```python
from build123d import *

# Parameters (mm, degrees)
F0_W     = 812.8
F0_H     = 2463.8
F1_DEPTH = 44.45
F3_D     = 228.6
F4_W     = 812.8
F4_H     = 50.8
F5_DEPTH = 3.429


# Not quite as in the source:
# - a feature names something its author has since deleted; it is built from what else it names


with BuildPart() as f1:
    # F0 (on Top) → F1 (new body)
    with BuildSketch(Plane.XY):
        with Locations((406.4, 1231.9)):
            Rectangle(F0_W, F0_H)
    extrude(amount=F1_DEPTH)

    # F3 (through all)
    with Locations(Plane.XY.offset(44.45)):
        with Locations((406.4, 1524)):
            Hole(F3_D / 2)

    # F4 (on face) → F5 (join)
    with BuildSketch(Plane.XY.offset(44.45)):
        with Locations((406.4, 2133.6)):
            Rectangle(F4_W, F4_H)
        with Locations((406.4, 2032)):
            Rectangle(F4_W, F4_H)
        with Locations((406.4, 1930.4)):
            Rectangle(F4_W, F4_H)
        with Locations((406.4, 1828.8)):
            Rectangle(F4_W, F4_H)
        with Locations((406.4, 1727.2)):
            Rectangle(F4_W, F4_H)
        with BuildLine():
            Line((0, 1549.4), (0, 1498.6))
            Line((0, 1498.6), (256.1315735093, 1498.6))
            ThreePointArc((256.1315735093, 1498.6), (254, 1524), (256.1315735093, 1549.4))
            Line((256.1315735093, 1549.4), (0, 1549.4))
        make_face()
        with BuildLine():
            Line((556.6684264907, 1498.6), (812.8, 1498.6))
            Line((812.8, 1498.6), (812.8, 1549.4))
            Line((812.8, 1549.4), (556.6684264907, 1549.4))
            ThreePointArc((556.6684264907, 1549.4), (558.2661716729, 1536.7446420666), (558.8, 1524))
            ThreePointArc((558.8, 1524), (558.2661716729, 1511.2553579334), (556.6684264907, 1498.6))
        make_face()
        with BuildLine():
            Line((490.642269675, 1397), (812.8, 1397))
            Line((812.8, 1397), (812.8, 1447.8))
            Line((812.8, 1447.8), (538.3822715367, 1447.8))
            ThreePointArc((538.3822715367, 1447.8), (517.455945611, 1419.6336407436), (490.642269675, 1397))
        make_face()
        with Locations((406.4, 1320.8)):
            Rectangle(F4_W, F4_H)
        Polygon((0, 1231.9), (0, 1193.8), (812.8, 1193.8), (812.8, 1231.9), (812.8, 1244.6), (0, 1244.6), align=None)
        with Locations((406.4, 1117.6)):
            Rectangle(F4_W, F4_H)
        with Locations((406.4, 1016)):
            Rectangle(F4_W, F4_H)
        with Locations((406.4, 914.4)):
            Rectangle(F4_W, F4_H)
        with Locations((406.4, 812.8)):
            Rectangle(F4_W, F4_H)
        with Locations((406.4, 711.2)):
            Rectangle(F4_W, F4_H)
        with Locations((406.4, 609.6)):
            Rectangle(F4_W, F4_H)
        with Locations((406.4, 508)):
            Rectangle(F4_W, F4_H)
        with Locations((406.4, 406.4)):
            Rectangle(F4_W, F4_H)
        with Locations((406.4, 304.8)):
            Rectangle(F4_W, F4_H)
        with Locations((406.4, 203.2)):
            Rectangle(F4_W, F4_H)
        with BuildLine():
            Line((538.3822715367, 1600.2), (812.8, 1600.2))
            Line((812.8, 1600.2), (812.8, 1651))
            Line((812.8, 1651), (490.642269675, 1651))
            ThreePointArc((490.642269675, 1651), (517.455945611, 1628.3663592564), (538.3822715367, 1600.2))
        make_face()
        with BuildLine():
            Line((0, 1447.8), (0, 1397))
            Line((0, 1397), (322.157730325, 1397))
            ThreePointArc((322.157730325, 1397), (295.344054389, 1419.6336407436), (274.4177284633, 1447.8))
            Line((274.4177284633, 1447.8), (0, 1447.8))
        make_face()
        with BuildLine():
            Line((0, 1651), (0, 1600.2))
            Line((0, 1600.2), (274.4177284633, 1600.2))
            ThreePointArc((274.4177284633, 1600.2), (295.344054389, 1628.3663592564), (322.157730325, 1651))
            Line((322.157730325, 1651), (0, 1651))
        make_face()
    extrude(amount=-F5_DEPTH)


solid = f1.part
```
Model file for the job. Use its own axes, mm. Give positions to 0.01 mm unless a question says otherwise; leave off trailing zeros. Write each loop counter-clockwise with the first axis right and the second up, starting at its lowest first coordinate (ties: lowest second). Pieces come first, ordered by that corner, then holes. Notation, with made-up numbers: M 6.5,78 L 43.5,78 A37 ccw 43.5,117 Z; hole C -12.5,-3 d1. An arc over 180 degrees is marked long. Use a Markdown table: item, result.
1) Cut at A-A (x = 406.4). List the corners of the cut face in (y, z).
Responses:
| item | result |
|---|---|
| outline | M 0,0 L 1409.7,0 L 1409.7,44.45 L 0,44.45 Z; M 1638.3,0 L 2463.8,0 L 2463.8,44.45 L 1638.3,44.45 Z |
2) Drill centre lines: line 1 (Y direction, x = 406, z = 14); line 2 (Y direction, x = 397.5, z = 6). Where is each one in solid material? Low to high. Write a range as from..to.
Responses:
| item | result |
|---|---|
| line 1 | y = 0..1409.7, 1638.3..2463.8 |
| line 2 | y = 0..1410.05, 1637.95..2463.8 |
3) Cut at C-C (z = 37). List the corners of the cut face in (x, y).
Responses:
| item | result |
|---|---|
| outline | M 0,0 L 812.8,0 L 812.8,2463.8 L 0,2463.8 Z; hole C 406.4,1524 d228.6 |
4) Cut at B-B (y = 1524). List the corners of the cut face in (x, z), and give its area (3 significant figures).
Responses:
| item | result |
|---|---|
| outline | M 0,0 L 292.1,0 L 292.1,44.45 L 0,44.45 Z; M 520.7,0 L 812.8,0 L 812.8,44.45 L 520.7,44.45 Z |
| area | 26,000 mm2 |
5) Pull direction X, two halves, no side cores. Call faces 1 (the cylindrical face through (520.59, 1529.03, 21.91)), 2 (the flat face through (401, 1249, 44.45)), 3 (the flat face through (0, 1215, 22)): +X half, -X half, draft (parallel to the pull), parting line (faces both ways), or undercut.
Responses:
| item | result |
|---|---|
| face 1 | undercut |
| face 2 | draft |
| face 3 | -X half |
